```python
from build123d import *

# Parameters (mm, degrees)
F2_R            = 6
F4_DEPTH        = 10
F5_DEPTH        = 10
F9_W            = 85.8580678701
F9_H            = 17.2091361135
F10_DEPTH       = 25
F11_R           = 5.99999
F14_D           = 5
F14_START       = 1.5278641
F14_START_2     = 1.5278642
F14_CBORE_D     = 8
F14_CBORE_DEPTH = 2


# Not quite as in the source:
# - a fillet or chamfer is up to 0.001 mm smaller than in the source, because OpenCascade refuses the exact size


with BuildPart() as f3:
    # F3: sweep along a path in F0
    with BuildLine(Plane.XY) as f3_path:
        ThreePointArc((-27.5, 12.5), (-18.6611652352, 8.8388347648), (-15, 0))
        ThreePointArc((-15, 0), (0, -15), (15, 0))
        ThreePointArc((15, 0), (18.6611652352, 8.8388347648), (27.5, 12.5))
    # F2 (on offset) → F3 (sweep)
    with BuildSketch(Plane.YZ.offset(-27.5)):
        with Locations((12.5, 0)):
            Circle(F2_R)
    sweep(path=f3_path.line)

    # F4 (add): a face of the model
    f4_faces = [f3.faces().sort_by_distance(p)[0] for p in [
        (27.5, 12.5, 0),
    ]]
    extrude(f4_faces, amount=F4_DEPTH)

    # F5 (add): a face of the model
    f5_faces = [f3.faces().sort_by_distance(p)[0] for p in [
        (-27.5, 12.5, 0),
    ]]
    extrude(f5_faces, amount=F5_DEPTH)

    # F9 (on offset) → F10 (cut)
    with BuildSketch(Plane.XY.offset(6)):
        with Locations((5.4290339351, 21.1045680568)):
            Rectangle(F9_W, F9_H)
    extrude(amount=-F10_DEPTH, mode=Mode.SUBTRACT)

    # F11 (radius 6 in the source; OpenCascade refuses exactly that, so slightly less here)
    f11_edges = [f3.edges().sort_by_distance(p)[0] for p in [
        (-37.5, 6.5, 0),
        (37.5, 6.5, 0),
    ]]
    fillet(f11_edges, radius=F11_R)

    # F14 (through all)
    # its depths count from where the whole tool has entered the part; down to there all is cleared
    with Locations(Plane.XZ.offset(-6.5)):
        with Locations((-31.5, 0, -F14_START), (31.5, 6.2e-09, -F14_START_2)):
            CounterBoreHole(F14_D / 2, F14_CBORE_D / 2, F14_CBORE_DEPTH)


solid = f3.part
```
Design review of the part built by this model. Coordinates are the model's own, in mm. A direction names the side the tool comes from. Coordinates: 2 decimals unless noted, no trailing zeros. Answer as a JSON object with one key per item and string values. Group by question number.
1) For pin 1 (4 mm diameter, centred on x = -31.5, z = 0, fed in from +Y); pin 2 (2 mm diameter, centred on x = 4, z = -3, fed in from +Y); pin 3 (3 mm diameter, centred on y = 8.5, z = 4, fed in from -X); pin 4 (6.5 mm diameter, centred on x = 30.5, z = -0.5, fed in from -Y), all flat-tipped, find the tip position at first contact; note any pin that passes through.
2) Mouldability with a two-part tool opening along Y and no side actions: class faces 4 (the cylindrical face through (27.504, 8.631, 0.176)), 5 (the cylindrical face through (-27.685, 8.631, 1.201)), 6 (the flat face through (26, 12.5, 0)), 7 (the cylindrical face through (29.472, 9.905, 5.41)) as pulls with the +Y half, pulls with the -Y half, needs draft (parallel to the pull), parting line crosses it, or undercut.
3) Wall thickness on L1, parallel to X at y = 11.5, z = -1; L2, parallel to Z at x = 31.5, y = 8.2; L3, parallel to Z at x = -14.5, y = -5: over which ranges is each line inside the solid? List them lowest first.
4) Add section A-A, the plane z = 1.5. Count the separate pieces of the cut face and the enclosed holes in it, then the cut area to 3 significant figures.
5) Tool access review of faces 1 (the cylindrical face through (-29.472, 9.905, 5.41)), 2 (the flat face through (-32, 10.028, -3)), 3 (the cylindrical face through (-29.47, 9.11, -4.95)): name each direction out of +Z, -Z, +X, -X, +Y, -Y from which nothing blocks a thin tool from reaching the whole face with its end or side.
Computed values:
{
 "1": {"pin 1": "passes through", "pin 2": "stops at y = -8.2", "pin 3": "stops at x = -35.83", "pin 4": "stops at y = 6.5"},
 "2": {"face 4": "undercut", "face 5": "undercut", "face 6": "pulls with the +Y half", "face 7": "pulls with the -Y half"},
 "3": {"L1": "x = -37.33 to -33.79, -29.21 to -13.12, 13.12 to 29.21, 33.79 to 37.33", "L2": "z = -4.18 to -4, 4 to 4.18", "L3": "z = -5.99 to 5.99"},
 "4": {"separate pieces": "3", "enclosed holes": "0", "area": "930 mm^2"},
 "5": {"face 1": "+Z, -X, -Y", "face 2": "-Y", "face 3": "-Z, -X, -Y"}
}
